Design review of the part built by this model. Coordinates are the model's own, in mm. Round coordinates to 2 decimals unless told otherwise and drop trailing zeros. Loops run counter-clockwise (first coordinate to the right, second up) from the corner with the lowest first, then second, coordinate; pieces in that order, holes last. Notation, with made-up numbers: (4, -38) - (17, -38) arc R33 ccw to (17, -3) - close; hole circle Ø1 at (71, -30.5). An arc over 180 degrees is marked (long way). Answer as CSV lines item,"result". Start each with the question number.
(1) Consider section C-C (x = 26). Give the boundary of the cut face in (y, z), and give its area (3 significant figures).
(2) Mouldability with a two-part tool opening along Z and no side actions: class faces 1 (the flat face through (-1, 1, 27.5)), 2 (the cylindrical face through (11.5, 1.5, -21.3)) as released by +Z, released by -Z, zero draft, split by the parting line, or undercut.
(3) For P1, Ø1.8, axis at x = 62.5, z = 18.3, coming from the +Y side, flat-tipped, find the tip position at first contact; note if it passes through.
(4) Consider section B-B (z = 11). Give the boundary of the cut face in (x, y), and give its area (3 significant figures).
(5) Consider section A-A (x = -62.5). Give the boundary of the cut face in (y, z), and give its area (3 significant figures).
(6) Consider section D-D (y = 0.7). Count the separate pieces of the cut face and the enclosed holes in it, and give its area (3 significant figures).
(7) Wall thickness on L1, parallel to Z at x = -49.5, y = 1.9; L2, parallel to X at y = 2.25, z = -18.3; L3, parallel to Z at x = 2.5, y = 2.65: over which ranges is each line inside the solid? List them lowest first.
from build123d import *

# Parameters (mm, degrees)
ESBO_O1_W                = 145
ESBO_O1_H                = 55
RESSALTO_EXTRUS_O1_DEPTH = 3
ESBO_O2_R                = 1.5
CORTE_EXTRUS_O1_DEPTH    = 3


with BuildPart() as part:
    # Esboço1 → Ressalto-extrusão1 (new body)
    with BuildSketch(Plane(origin=(0, 0, 0), x_dir=(1, 0, 0), z_dir=(0, 1, 0))):
        Rectangle(ESBO_O1_W, ESBO_O1_H)
    extrude(amount=RESSALTO_EXTRUS_O1_DEPTH)

    # Esboço2 → Corte-extrusão1 (cut)
    with BuildSketch(Plane(origin=(0, 3, 0), x_dir=(1, 0, 0), z_dir=(0, 1, 0))):
        with Locations(Location((-62.5, 18.3, 0), (0, 0, 270))):
            Circle(ESBO_O2_R)
        with Locations(Location((-62.5, -18.3, 0), (0, 0, 90))):
            Circle(ESBO_O2_R)
        with Locations(Location((62.5, -18.3, 0), (0, 0, 270))):
            Circle(ESBO_O2_R)
        with Locations(Location((62.5, 18.3, 0), (0, 0, 90))):
            Circle(ESBO_O2_R)
        with BuildLine():
            Line((-10.25, 22.5), (10.25, 22.5))
            ThreePointArc((10.25, 22.5), (11.5, 21.25), (10.25, 20))
            Line((10.25, 20), (-10.25, 20))
            ThreePointArc((-10.25, 20), (-11.5, 21.25), (-10.25, 22.5))
        make_face()
        with BuildLine():
            Line((-50, 12.5), (50, 12.5))
            ThreePointArc((50, 12.5), (51.5, 11), (50, 9.5))
            Line((50, 9.5), (-50, 9.5))
            ThreePointArc((-50, 9.5), (-51.5, 11), (-50, 12.5))
        make_face()
        with BuildLine():
            Line((-10.25, -22.5), (10.25, -22.5))
            ThreePointArc((10.25, -22.5), (11.5, -21.25), (10.25, -20))
            Line((10.25, -20), (-10.25, -20))
            ThreePointArc((-10.25, -20), (-11.5, -21.25), (-10.25, -22.5))
        make_face()
        with BuildLine():
            Line((-50, -12.5), (50, -12.5))
            ThreePointArc((50, -12.5), (51.5, -11), (50, -9.5))
            Line((50, -9.5), (-50, -9.5))
            ThreePointArc((-50, -9.5), (-51.5, -11), (-50, -12.5))
        make_face()
        with BuildLine():
            Line((-50, 1.5), (50, 1.5))
            ThreePointArc((50, 1.5), (51.5, 0), (50, -1.5))
            Line((50, -1.5), (-50, -1.5))
            ThreePointArc((-50, -1.5), (-51.5, 0), (-50, 1.5))
        make_face()
    extrude(amount=-CORTE_EXTRUS_O1_DEPTH, mode=Mode.SUBTRACT)


solid = part.part
Determined:
1,outline,"(0, -27.5) - (3, -27.5) - (3, -12.5) - (0, -12.5) - close; (0, -9.5) - (3, -9.5) - (3, -1.5) - (0, -1.5) - close; (0, 1.5) - (3, 1.5) - (3, 9.5) - (0, 9.5) - close; (0, 12.5) - (3, 12.5) - (3, 27.5) - (0, 27.5) - close"
1,area,"138 mm^2"
2,face 1,"released by +Z"
2,face 2,"undercut"
3,P1,"passes through"
4,outline,"(-72.5, 0) - (-51.5, 0) - (-51.5, 3) - (-72.5, 3) - close; (51.5, 0) - (72.5, 0) - (72.5, 3) - (51.5, 3) - close"
4,area,"126 mm^2"
5,outline,"(0, -27.5) - (3, -27.5) - (3, -19.8) - (0, -19.8) - close; (0, -16.8) - (3, -16.8) - (3, 16.8) - (0, 16.8) - close; (0, 19.8) - (3, 19.8) - (3, 27.5) - (0, 27.5) - close"
5,area,"147 mm^2"
6,separate pieces,"1"
6,enclosed holes,"9"
6,area,"6,910 mm^2"
7,L1,"z = -27.5 to -12.5, -9.5 to -1.5, 1.5 to 9.5, 12.5 to 27.5"
7,L2,"x = -72.5 to -64, -61 to 61, 64 to 72.5"
7,L3,"z = -27.5 to -22.5, -20 to -12.5, -9.5 to -1.5, 1.5 to 9.5, 12.5 to 20, 22.5 to 27.5"
